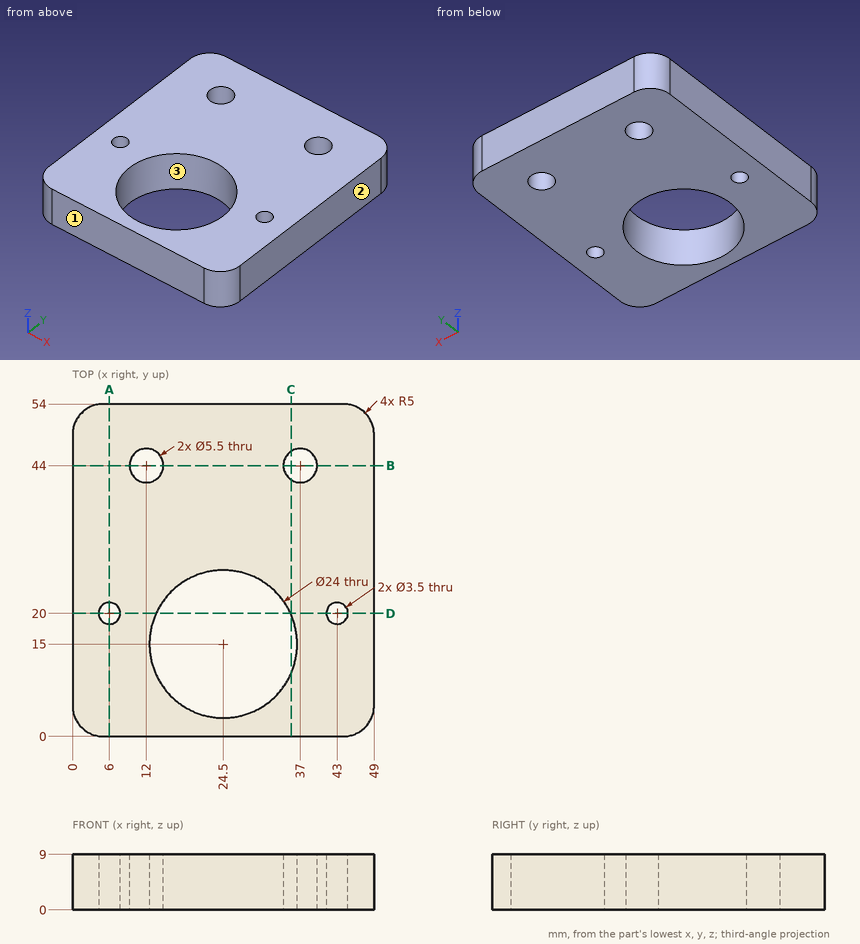
Print and shaded views of the part. All mm, measured from the part's lowest x, y and z. Coordinates: 2 decimals unless noted, no trailing zeros. Order: outer loops, then holes, each group sorted by start corner. A loop starts at its lowest first (then second) coordinate and runs counter-clockwise, first axis right, second up.
(1) Probe L1, parallel to Y at x = 37, z = 7.25; L2, parallel to Y at x = 6, z = 3.25; L3, parallel to Y at x = 34.5, z = 5. List the from-to ranges inside material, lowest first.
Check sheet entries:
L1: y = 0 to 41.25, 46.75 to 54
L2: y = 0 to 18.25, 21.75 to 54
L3: y = 0 to 8.37, 21.63 to 42.85, 45.15 to 54
(2) Pull direction Y, two halves, no side cores. Call the marked faces 1, 2 and 3: pulls with the +Y half, pulls with the -Y half, needs draft (parallel to the pull), parting line crosses it, or undercut.
Check sheet entries:
face 1: pulls with the -Y half
face 2: needs draft
face 3: undercut
(3) Slice it at C-C, the plane x = 35.5. Write the cut outline in (y, z).
Check sheet entries:
outline: (0, 0) - (10.2, 0) - (10.2, 9) - (0, 9) - close; (19.8, 0) - (41.7, 0) - (41.7, 9) - (19.8, 9) - close; (46.3, 0) - (54, 0) - (54, 9) - (46.3, 9) - close
(4) Slice it at D-D, the plane y = 20. Write the cut outline in (x, z), and give its area (3 significant figures).
Check sheet entries:
outline: (0, 0) - (4.25, 0) - (4.25, 9) - (0, 9) - close; (7.75, 0) - (13.59, 0) - (13.59, 9) - (7.75, 9) - close; (35.41, 0) - (41.25, 0) - (41.25, 9) - (35.41, 9) - close; (44.75, 0) - (49, 0) - (49, 9) - (44.75, 9) - close
area: 182 mm2
(5) Pin check, flat tips, straight feed: pin 1 Ø3 at (x, y) = (6, 20) entering from -Z; pin 2 Ø2 at (x, y) = (21.5, 30.5) entering from -Z. Stop position of each tip, or through.
Check sheet entries:
pin 1: passes through
pin 2: stops at z = 0
(6) Slice it at B-B, the plane y = 44. Write the cut outline in (x, z), and give its area (3 significant figures).
Check sheet entries:
outline: (0, 0) - (9.25, 0) - (9.25, 9) - (0, 9) - close; (14.75, 0) - (34.25, 0) - (34.25, 9) - (14.75, 9) - close; (39.75, 0) - (49, 0) - (49, 9) - (39.75, 9) - close
area: 342 mm2
(7) Slice it at A-A, the plane x = 6. Write the cut outline in (y, z), and give its area (4 significant figures).
Check sheet entries:
outline: (0, 0) - (18.25, 0) - (18.25, 9) - (0, 9) - close; (21.75, 0) - (54, 0) - (54, 9) - (21.75, 9) - close
area: 454.5 mm2
